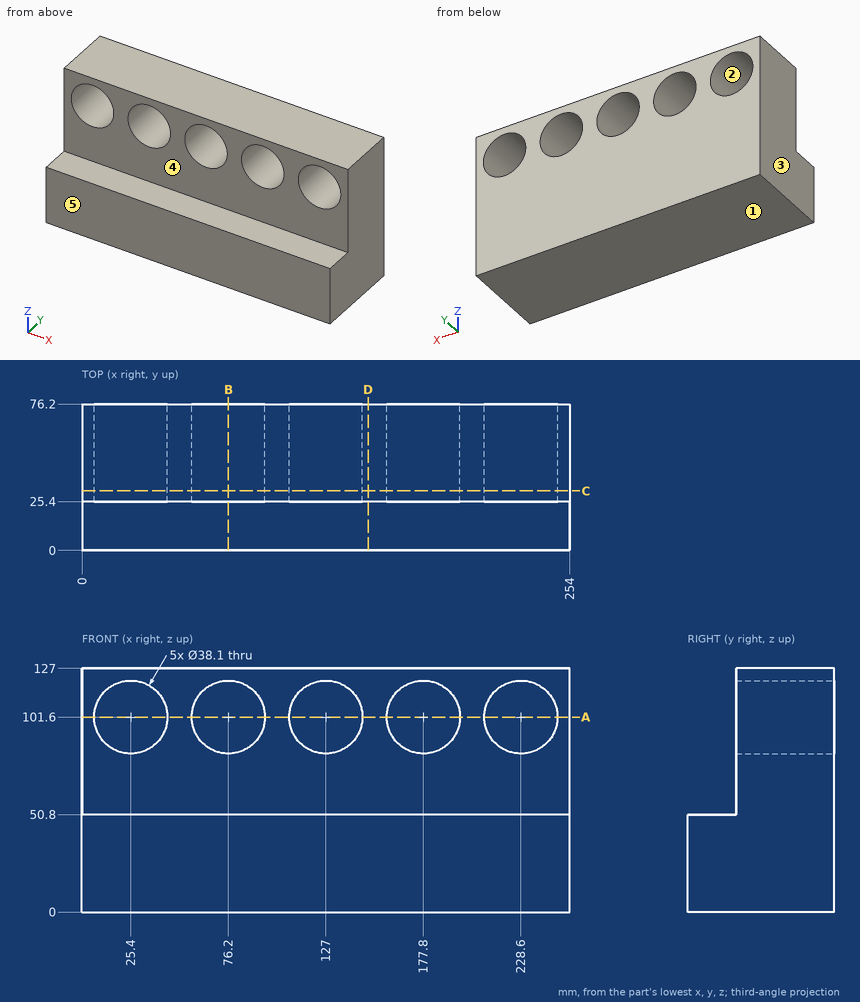
Geometry check sheet. Reference: drawing and pictorial views, mm from the part's lowest x, y, z. A direction names the side the tool comes from. Give positions to 0.01 mm unless a question says otherwise; leave off trailing zeros. Write each loop counter-clockwise with the first axis right and the second up, starting at its lowest first coordinate (ties: lowest second). Pieces come first, ordered by that corner, then holes.
Item 1: Cross-section at A-A (z = 101.6). Enter the section's corners in (x, y), and give its area (3 significant figures).
Item 2: Access from +Z, -Z, +X, -X, +Y, -Y to the whole of each face (thin tool, end or side, straight path). Record for the marked faces 4 and 5.
Item 3: Scan lines: L1, parallel to X at y = 66, z = 101; L2, parallel to Z at x = 25, y = 49; L3, parallel to X at y = 57.5, z = 108. Record each from-to range of solid material in increasing order.
Item 4: Cross-section at B-B (x = 76.2). Enter the section's corners in (y, z), and give its area (3 significant figures).
Item 5: Cross-section at C-C (y = 31). Enter the section's corners in (x, z), and give its area (3 significant figures).
Item 6: Gauge pin test, flat ends, axial feed: pin 1 (23 mm diameter, centred on x = 177.8, z = 101.6, fed in from +Y); pin 2 (23 mm diameter, centred on x = 90, z = 105.5, fed in from -Y); pin 3 (20.5 mm diameter, centred on x = 99, y = 11.5, fed in from +Z). Record the tip position at first contact, or that the pin passes through.
Item 7: Cross-section at D-D (x = 149). Enter the section's corners in (y, z), and give its area (3 significant figures).
Item 8: Draft check along X on the marked faces 1, 2 and 3. Enter one of: released by +X, released by -X, zero draft, split by the parting line, or undercut.
Report:
1. outline: (0, 25.4) - (6.35, 25.4) - (6.35, 76.2) - (0, 76.2) - close; (44.45, 25.4) - (57.15, 25.4) - (57.15, 76.2) - (44.45, 76.2) - close; (95.25, 25.4) - (107.95, 25.4) - (107.95, 76.2) - (95.25, 76.2) - close; (146.05, 25.4) - (158.75, 25.4) - (158.75, 76.2) - (146.05, 76.2) - close; (196.85, 25.4) - (209.55, 25.4) - (209.55, 76.2) - (196.85, 76.2) - close; (247.65, 25.4) - (254, 25.4) - (254, 76.2) - (247.65, 76.2) - close
1. area: 3,230 mm2
2. face 4: +Z, +X, -X, -Y
2. face 5: +Z, -Z, +X, -X, -Y
3. L1: x = 0 to 6.36, 44.44 to 57.16, 95.24 to 107.96, 146.04 to 158.76, 196.84 to 209.56, 247.64 to 254
3. L2: z = 0 to 82.55, 120.65 to 127
3. L3: x = 0 to 7.46, 43.34 to 58.26, 94.14 to 109.06, 144.94 to 159.86, 195.74 to 210.66, 246.54 to 254
4. outline: (0, 0) - (76.2, 0) - (76.2, 82.55) - (25.4, 82.55) - (25.4, 50.8) - (0, 50.8) - close; (25.4, 120.65) - (76.2, 120.65) - (76.2, 127) - (25.4, 127) - close
4. area: 5,810 mm2
5. outline: (0, 0) - (254, 0) - (254, 127) - (0, 127) - close; hole circle Ø38.1 at (25.4, 101.6); hole circle Ø38.1 at (76.2, 101.6); hole circle Ø38.1 at (127, 101.6); hole circle Ø38.1 at (177.8, 101.6); hole circle Ø38.1 at (228.6, 101.6)
5. area: 26,600 mm2
6. pin 1: passes through
6. pin 2: stops at y = 25.4
6. pin 3: stops at z = 50.8
7. outline: (0, 0) - (76.2, 0) - (76.2, 127) - (25.4, 127) - (25.4, 50.8) - (0, 50.8) - close
7. area: 7,740 mm2
8. face 1: zero draft
8. face 2: undercut
8. face 3: released by -X
